Geometry: final body of the model. Coordinates: model frame, mm. Face numbers are marked on the shaded views. A direction names the side the tool comes from. Give positions to 0.01 mm unless a question says otherwise; leave off trailing zeros. Loops run counter-clockwise (first coordinate to the right, second up) from the corner with the lowest first, then second, coordinate; pieces in that order, holes last.
```python
from build123d import *

# Parameters (mm, degrees)
EXTRUDE_1_DEPTH               = 60
SKETCH_2_R                    = 3
CUT_EXTRUDE_1_DEPTH           = 83.791703555
HOLE_WIZARD_M10_1_D           = 8.5
HOLE_WIZARD_M10_1_DEPTH       = 27.5
HOLE_WIZARD_M10_1_CSINK_D     = 11.05
HOLE_WIZARD_M10_1_CSINK_ANGLE = 90
HOLE_WIZARD_M10_1_TIP         = 2.553657631


with BuildPart() as part:
    # 草图1 → 凸台-拉伸1 (new body)
    with BuildSketch(Plane.XY):
        with BuildLine():
            Line((-34.31692533, -27.181035016), (-34.31692533, 32.818964984))
            Line((-34.31692533, 32.818964984), (-28.31692533, 32.818964984))
            Line((-28.31692533, 32.818964984), (-28.31692533, 13.062622536))
            ThreePointArc((-28.31692533, 13.062622536), (-11.291229121, 20.680947179), (3.345497613, 9.118964984))
            Line((3.345497613, 9.118964984), (18.345497613, 9.118964984))
            Line((18.345497613, 9.118964984), (18.345497613, 3.118964984))
            Line((18.345497613, 3.118964984), (-1.519747569, 3.118964984))
            ThreePointArc((-1.519747569, 3.118964984), (-25.515996982, 2.818964984), (-1.519747569, 2.518964984))
            Line((-1.519747569, 2.518964984), (18.345497613, 2.518964984))
            Line((18.345497613, 2.518964984), (18.345497613, -3.481035016))
            Line((18.345497613, -3.481035016), (3.345497613, -3.481035016))
            ThreePointArc((3.345497613, -3.481035016), (-11.291229121, -15.043017212), (-28.31692533, -7.424692569))
            Line((-28.31692533, -7.424692569), (-28.31692533, -27.181035016))
            Line((-28.31692533, -27.181035016), (-34.31692533, -27.181035016))
        make_face()
    extrude(amount=EXTRUDE_1_DEPTH)

    # 草图2 → 切除-拉伸1 (cut, through all)
    with BuildSketch(Plane(origin=(-28.31692533, 0, 0), x_dir=(0, 0, -1), z_dir=(1, 0, 0))):
        with Locations((-45, 25.318964984)):
            Circle(SKETCH_2_R)
        with Locations((-15, 25.318964984)):
            Circle(SKETCH_2_R)
    cut_extrude_1 = extrude(amount=-CUT_EXTRUDE_1_DEPTH, mode=Mode.SUBTRACT)

    # 镜向3: 切除-拉伸1 across plane
    add(cut_extrude_1.mirror(Plane.ZX.offset(2.818964984)), mode=Mode.SUBTRACT)

    # M10 螺纹孔1
    with Locations(Plane(origin=(10.845497613, 9.118964984, 15), x_dir=(1, 0, 0), z_dir=(0, 1, 0))):
        with Locations((0, 0), (0, -30)):
            CounterSinkHole(HOLE_WIZARD_M10_1_D / 2, HOLE_WIZARD_M10_1_CSINK_D / 2, depth=HOLE_WIZARD_M10_1_DEPTH, counter_sink_angle=HOLE_WIZARD_M10_1_CSINK_ANGLE)
            with Locations((0, 0, -(HOLE_WIZARD_M10_1_DEPTH + HOLE_WIZARD_M10_1_TIP / 2))):  # 118° drill point
                Cone(0, HOLE_WIZARD_M10_1_D / 2, HOLE_WIZARD_M10_1_TIP, mode=Mode.SUBTRACT)


solid = part.part
```
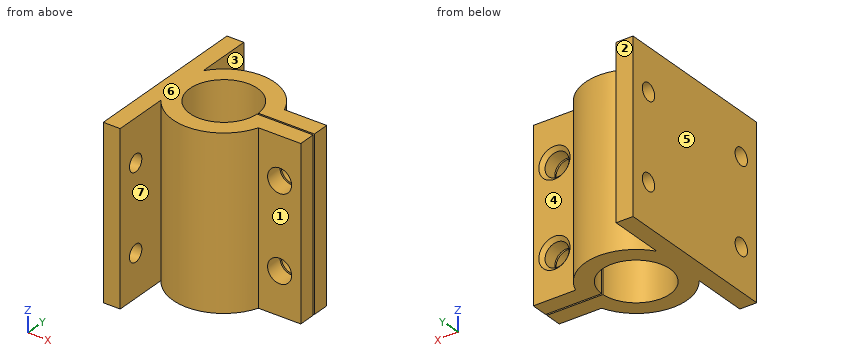
Q1. Reachability of the marked faces 1, 2, 3 and 4 from +Z, -Z, +X, -X, +Y, -Y: full face, straight path, thin tool, end or side. Return the list, or none.
Q2. Mould query, pull axis X, two halves, no side actions, for the marked faces 5, 6 and 7. Classes: +X half, -X half, draft (parallel to the pull), parting line (faces both ways), or undercut.
Q3. Material intervals for probe 1 along Y at (x, z) = (-30, 45); probe 2 along X at (y, z) = (-20.5, 23); probe 3 along X at (y, z) = (6.5, 17.5), sorted ascending.
Q4. Section query A-A, the plane z = 15. State how many separate pieces and enclosed holes the cut face has, and give its area (3 significant figures).
Q5. Section query D-D, the plane x = -13. Return loops of the section in (y, z).
Q6. Section query B-B, the plane z = 28. Return loops of the section in (x, y), and give its area (3 significant figures).
Q7. Pin query (flat end, axial travel): pin 1 Ø4.5 at (x, z) = (12, 24.5) entering from +Y; pin 2 Ø1 at (y, z) = (-16.5, 12) entering from +X; pin 3 Ø12 at (x, z) = (13, 20) entering from -Y. Return the tip coordinate at first contact, or that it passes through.
Q8. Section query C-C, the plane x = -31. Return loops of the section in (y, z), and give its area (3 significant figures).
Resolved:
1. face 1: +Z, -Z, +X, -Y
1. face 2: +Z, -Z, +X, -X, +Y
1. face 3: +Z, -Z, +Y
1. face 4: +Z, -Z, +X, +Y
2. face 5: -X half
2. face 6: draft
2. face 7: undercut
3. probe 1: y = -27.18 to -22.68, -16.68 to 22.32, 28.32 to 32.82
3. probe 2: x = -34.32 to -28.32
3. probe 3: x = -34.32 to -24.94, -2.09 to 7.41, 14.28 to 18.35
4. separate pieces: 5
4. enclosed holes: 0
4. area: 873 mm2
5. outline: (-15.17, 0) - (-9.17, 0) - (-9.17, 60) - (-15.17, 60) - close; (14.81, 0) - (20.81, 0) - (20.81, 60) - (14.81, 60) - close
6. outline: (-34.32, -27.18) - (-28.32, -27.18) - (-28.32, -7.42) arc R18 ccw to (3.35, -3.48) - (18.35, -3.48) - (18.35, 2.52) - (-1.52, 2.52) arc R12 cw (long way) to (-1.52, 3.12) - (18.35, 3.12) - (18.35, 9.12) - (3.35, 9.12) arc R18 ccw to (-28.32, 13.06) - (-28.32, 32.82) - (-34.32, 32.82) - close
6. area: 1,050 mm2
7. pin 1: stops at y = 9.12
7. pin 2: stops at x = -28.32
7. pin 3: stops at y = -3.48
8. outline: (-27.18, 0) - (32.82, 0) - (32.82, 60) - (-27.18, 60) - close; hole circle Ø6 at (-19.68, 15); hole circle Ø6 at (-19.68, 45); hole circle Ø6 at (25.32, 15); hole circle Ø6 at (25.32, 45)
8. area: 3,490 mm2
